from build123d import *

# Parameters (mm, degrees)
F0_W     = 400
F0_H     = 600
F1_DEPTH = 110
F2_W     = 220
F2_H     = 100
F2_H_2   = 177.977299
F3_DEPTH = 600.001
F4_W     = 200
F4_H     = 90
F5_DEPTH = 401
F6_W     = 380
F6_H     = 580
F7_DEPTH = 850


with BuildPart() as f1:
    # F0 (on Top) → F1 (new body)
    with BuildSketch(Plane.XY):
        with Locations((-45.659611, 95.696688)):
            Rectangle(F0_W, F0_H)
    extrude(amount=F1_DEPTH)

    # F2 (on face) → F3 (cut, through all)
    with BuildSketch(Plane.XZ.offset(204.303312)):
        with Locations((-45.659611, 50)):
            Rectangle(F2_W, F2_H)
        with Locations((-45.659611, -88.988649)):
            Rectangle(F2_W, F2_H_2)
    extrude(amount=-F3_DEPTH, mode=Mode.SUBTRACT)

    # F4 (on face) → F5 (cut)
    with BuildSketch(Plane(origin=(-245.659611, 0, 0), x_dir=(0, -1, 0), z_dir=(-1, 0, 0))):
        with Locations((-95.696688, 55)):
            Rectangle(F4_W, F4_H)
    extrude(amount=-F5_DEPTH, mode=Mode.SUBTRACT)

    # F6 (on face) → F7 (join)
    with BuildSketch(Plane.XY.offset(110)):
        with Locations((-45.659611, 95.696688)):
            Rectangle(F6_W, F6_H)
    extrude(amount=F7_DEPTH)


solid = f1.part
Here's how the part is built. I have some questions about the finished solid (model axes, mm). A direction names the side the tool comes from. Coordinates: 2 decimals unless noted, no trailing zeros. Loops run counter-clockwise (first coordinate to the right, second up) from the corner with the lowest first, then second, coordinate; pieces in that order, holes last.
1. Imagine slicing it at C-C, the plane x = 104.5. Please give me the cut outline in (y, z).
2. For faces 1 (the flat face through (-48, 100, 100)), 2 (the flat face through (-48, 385.697, 529)), 3 (the flat face through (109, 195.697, 54)), which set-ups out of +Z, -Z, +X, -X, +Y, -Y let a thin tool reach every point of the face, with its end or its side?
3. Imagine slicing it at B-B, the plane z = 58.5. Please give me the cut outline in (x, y), and give its area (3 significant figures).
4. Imagine slicing it at D-D, the plane x = -46.5. Please give me the cut outline in (y, z), and give its area (3 significant figures).
5. If we mould it in two halves opening along Y, with no side actions, what happens to faces 4 (the flat face through (-48, -194.303, 529)), 5 (the flat face through (-201, 97, 10)), 6 (the flat face through (-155.66, 91, 6))? For each: pulls with the +Y half, pulls with the -Y half, needs draft (parallel to the pull), parting line crosses it, or undercut.
6. For P1, Ø1, axis at x = -120.5, y = 39, coming from the -Z side; P2, Ø4, axis at x = 70, z = 231, coming from the +Y side; P3, Ø6, axis at x = -173, z = 343.5, coming from the -Y side, each with a flat end and sliding along its axis, tell me the tip position at first contact or that it passes through.
7. Imagine slicing it at A-A, the plane y = 166.5. Please give me the cut outline in (x, z).
8. I need wall thicknesses on L1, parallel to Z at x = 127.5, y = 18; L2, parallel to X at y = 266.5, z = 483; L3, parallel to Y at x = 112, z = 714.5. Which ranges of each line are inside material? Lowest first, please.
Taken from the geometry:
1. outline: (-204.3, 0) - (395.7, 0) - (395.7, 110) - (385.7, 110) - (385.7, 960) - (-194.3, 960) - (-194.3, 110) - (-204.3, 110) - close; hole (-4.3, 10) - (195.7, 10) - (195.7, 100) - (-4.3, 100) - close
2. face 1: none
2. face 2: +Z, +X, -X, +Y
2. face 3: +X, -X
3. outline: (-245.66, -204.3) - (-155.66, -204.3) - (-155.66, -4.3) - (-245.66, -4.3) - close; (-245.66, 195.7) - (-155.66, 195.7) - (-155.66, 395.7) - (-245.66, 395.7) - close; (64.34, -204.3) - (154.34, -204.3) - (154.34, -4.3) - (64.34, -4.3) - close; (64.34, 195.7) - (154.34, 195.7) - (154.34, 395.7) - (64.34, 395.7) - close
3. area: 72,000 mm2
4. outline: (-204.3, 100) - (395.7, 100) - (395.7, 110) - (385.7, 110) - (385.7, 960) - (-194.3, 960) - (-194.3, 110) - (-204.3, 110) - close
4. area: 499,000 mm2
5. face 4: pulls with the -Y half
5. face 5: undercut
5. face 6: needs draft
6. P1: stops at z = 100
6. P2: stops at y = 385.7
6. P3: stops at y = -194.3
7. outline: (-245.66, 0) - (-155.66, 0) - (-155.66, 10) - (-245.66, 10) - close; (-245.66, 100) - (154.34, 100) - (154.34, 110) - (144.34, 110) - (144.34, 960) - (-235.66, 960) - (-235.66, 110) - (-245.66, 110) - close; (64.34, 0) - (154.34, 0) - (154.34, 10) - (64.34, 10) - close
8. L1: z = 0 to 10, 100 to 960
8. L2: x = -235.66 to 144.34
8. L3: y = -194.3 to 385.7
